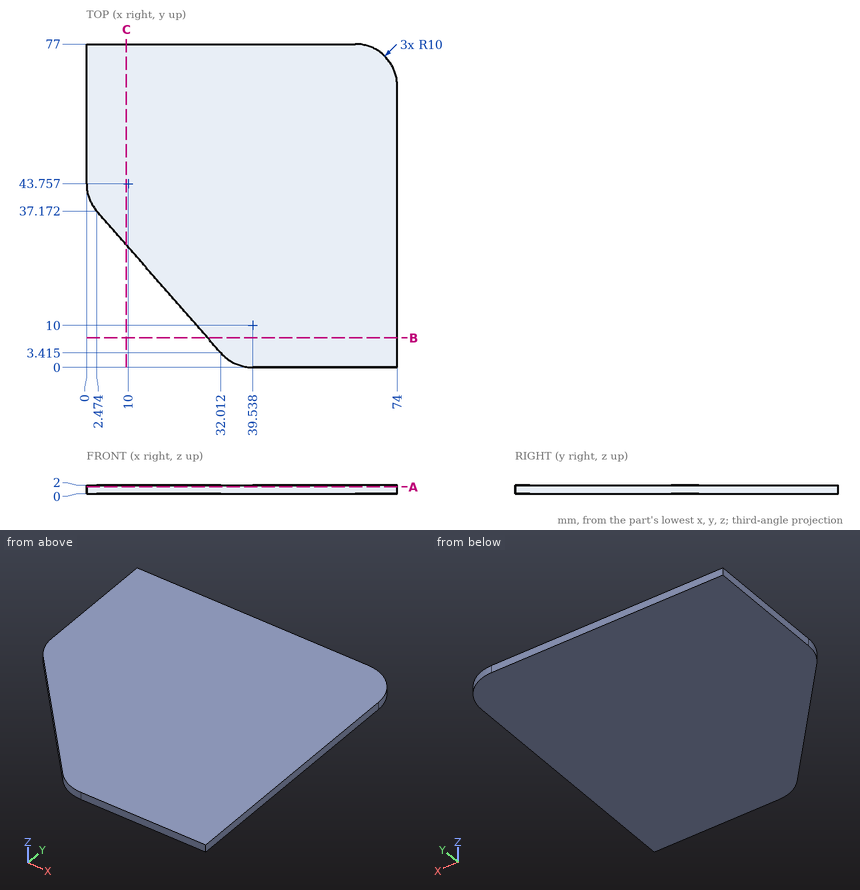
The figure shows three views and two pictorial views of one solid part (mm, origin at its lowest corner). Answer the questions. Round coordinates to 2 decimals unless told otherwise and drop trailing zeros. Loops run counter-clockwise (first coordinate to the right, second up) from the corner with the lowest first, then second, coordinate; pieces in that order, holes last. Notation, with made-up numbers: M 38.25,45 L 71.25,45 A13 ccw 71.25,66 Z; hole C -14.75,45.25 d3. An arc over 180 degrees is marked long. Use CSV: the item, a comma, the result in double quotes.
Q1. Section B-B, the plane y = 7 is taken. Determine the outline of the cut face in (x, z) (1 decimal).
Determined:
outline,"M 28.9,0 L 74,0 L 74,2 L 28.9,2 Z"
Q2. Section C-C, the plane x = 9.5 is taken. Determine the outline of the cut face in (y, z).
Determined:
outline,"M 29.14,0 L 77,0 L 77,2 L 29.14,2 Z"
Q3. This flat-tipped pin is pushed along its axis until it touches: pin 1 (5 mm diameter, centred on x = 61.5, y = 69, fed in from -Z). Where does it stop, or does it pass through?
Determined:
pin 1,"z = 0"
Q4. Consider L1, parallel to Y at x = 7, z = 1.15; L2, parallel to Y at x = 4, z = 0.6; L3, parallel to X at y = 17.5, z = 1.15. Determine where each line is inside the solid, lowest interval first.
Determined:
L1,"32 to 77"
L2,"35.43 to 77"
L3,"19.69 to 74"
Q5. Section A-A, the plane z = 1.6 is taken. Determine the outline of the cut face in (x, y) (1 decimal), then the cut area to 3 significant figures.
Determined:
outline,"M 0,43.8 A10 ccw 2.5,37.2 L 32,3.4 A10 ccw 39.5,0 L 74,0 L 74,67 A10 ccw 64,77 L 0,77 Z"
area,"4,970 mm2"
